Autodesk Inventor part; units mm, degrees
sketch "Sketch1" plane through (0, 0, 0) normal (0, 0, 1) x (1, 0, 0)
  line L0 (-109.5, 84.5) -> (109.5, 84.5)
  line L1 (109.5, 84.5) -> (109.5, -84.5)
  line L2 (109.5, -84.5) -> (-109.5, -84.5)
  line L3 (-109.5, -84.5) -> (-109.5, 84.5)
  point P0 (0, 84.5)
  point P1 (0, 0)
  point P2 (-109.5, 0)
  dimension "d0" = 219
  dimension "d1" = 169
extrude "Extrusion1" add sketch "Sketch1" along normal blind 6
sketch "Sketch2" plane through (0, 0, 6) normal (0, 0, 1) x (1, 0, 0)
  circle A0 centre (-103, -78) radius 3.25
  line L0 (-103, -78) -> (-103, -74) construction
  line L1 (-106.25, -68) -> (-99.75, -68)
  line L2 (-99.75, -68) -> (-99.75, -74)
  line L3 (-99.75, -74) -> (-106.25, -74)
  line L4 (-106.25, -74) -> (-106.25, -68)
  line L5 (-109.5, -84.5) -> (109.5, -84.5)
  line L6 (-109.5, -84.5) -> (-103, -84.5) construction
  line L7 (-103, -84.5) -> (-103, -78) construction
  point P0 (0, 0)
  dimension "d39" = 6.5
  dimension "d44" = 4
  dimension "d45" = 6.5
  dimension "d46" = 6
  dimension "d64" = 6.5
  dimension "d65" = 6.5
extrude "Extrusion2" cut sketch "Sketch2" against normal blind 6 contours A0
mirror "Mirror3" about plane through (0, 0, 0) normal (1, 0, 0) of "Extrusion2"
mirror "Mirror7" about plane through (0, 0, 0) normal (0, 1, 0) of "Extrusion2", "Mirror3"
sketch "Sketch7" plane through (0, 0, 6) normal (0, 0, 1) x (1, 0, 0)
  line L0 (-109.5, 84.5) -> (-109.5, -84.5)
  line L1 (-109.5, 68) -> (-75, 68)
  line L2 (-75, 68) -> (-75, -68)
  line L3 (-75, -68) -> (-109.5, -68)
  line L4 (-109.5, -68) -> (-109.5, 68)
  point P0 (0, 0)
  point P1 (-109.5, 0)
  point P2 (-109.5, 0)
  dimension "d40" = 34.5
  dimension "d41" = 136
extrude "Extrusion6" cut sketch "Sketch7" against normal blind 10
sketch "Sketch8" plane through (0, 0, 6) normal (0, 0, 1) x (1, 0, 0)
  circle A0 centre (-103, -78) radius 3.25
  line L0 (-103, -78) -> (-103, -73.75) construction
  line L1 (-106.125, -68) -> (-99.875, -68)
  line L2 (-99.875, -68) -> (-99.875, -73.75)
  line L3 (-99.875, -73.75) -> (-106.125, -73.75)
  line L4 (-106.125, -73.75) -> (-106.125, -68)
  point P0 (0, 0)
  dimension "d47" = 4.25
  dimension "d48" = 6.25
  dimension "d49" = 5.75
extrude "Extrusion7" cut sketch "Sketch8" against normal blind 6 contours L1 L2 L3 L4
mirror "Mirror8" about plane through (0, 0, 0) normal (0, 1, 0) of "Extrusion7"
fillet "Fillet5" radius 1 12 edges at (-109.5, -84.5, 3) (109.5, -84.5, 3) (-75, -68, 3) (109.5, 84.5, 3) (-109.5, 84.5, 3) (-109.5, 68, 3) (-75, 68, 3) (-99.875, 68, 3) (-106.125, 68, 3) (-99.875, -68, 3) (-109.5, -68, 3) (-106.125, -68, 3)
sketch "Sketch10" plane through (0, 0, 6) normal (0, 0, 1) x (1, 0, 0)
  line L0 (-75, 44.5) -> (39, 44.5) construction
  line L1 (39, 44.5) -> (39, -44.5) construction
  line L2 (39, -44.5) -> (-75, -44.5) construction
  line L3 (-75, -44.5) -> (-75, 44.5) construction
  line L4 (-75, 67) -> (-75, -67)
  line L5 (-75, 44.5) -> (39, -44.5) construction
  circle A0 centre (0, 0) radius 8.25
  line L6 (0, 0) -> (0, 25) construction
  circle A1 centre (0, 25) radius 8.25
  point P0 (-75, 0)
  point P1 (-75, 0)
  point P2 (-75, 0)
  dimension "d53" = 114
  dimension "d54" = 89
  dimension "d55" = 16.5
  dimension "d56" = 25
  dimension "d57" = 16.5
extrude "Extrusion8" cut sketch "Sketch10" against normal through all
pattern_circular "Circular Pattern1" count 8 over 360 about axis through (0, 0, 6) along (0, 0, -1) of "Extrusion8"
equation "\"d7\" = d46"
properties part number "MDF_Top_Big_Mic" material "MDF Medium Density Fiberboard"
Read the model definition and answer for the solid it produces. Units are mm, in the model's axes. A direction names the side the tool comes from. Coordinates: 2 decimals unless noted, no trailing zeros. Loops run counter-clockwise (first coordinate to the right, second up) from the corner with the lowest first, then second, coordinate; pieces in that order, holes last. Notation, with made-up numbers: (-2, 71.5) - (17, 71.5) arc R25 ccw to (17, 98.5) - close; hole circle Ø11 at (34.5, -31). An arc over 180 degrees is marked (long way). Answer in a Markdown table with one row per item.
1. Straight lines are drawn through the part: line 1 (Y direction, x = 0, z = 3.95); line 2 (X direction, y = 0.5, z = 2.7); line 3 (X direction, y = 11, z = 1.7). For each, find the intervals that lie inside material, in ascending order.
Conclusion:
| item | result |
|---|---|
| line 1 | y = -84.5 to -33.25, -16.75 to -8.25, 8.25 to 16.75, 33.25 to 84.5 |
| line 2 | x = -75 to -33.23, -16.77 to -8.23, 8.23 to 16.77, 33.23 to 109.5 |
| line 3 | x = -75 to -22.52, -12.83 to 12.83, 22.52 to 109.5 |
2. Given pin 1 (6 mm diameter, centred on x = 103, y = 78, fed in from +Z); pin 2 (1.8 mm diameter, centred on y = -6, z = 4.5, fed in from -X), each flat-ended and moving along its own axis, determine where each tip first touches the part or whether it passes through.
Conclusion:
| item | result |
|---|---|
| pin 1 | passes through |
| pin 2 | stops at x = -75 |
3. Determine the mould class of faces 4 (the face through (-2, 39, 6)), 5 (the face through (-99.875, 71, 3)), 6 (the face through (109.5, 1, 3)) for opening direction X: +X half, -X half, draft (parallel to the pull), parting line (faces both ways), or undercut.
Conclusion:
| item | result |
|---|---|
| face 4 | draft |
| face 5 | undercut |
| face 6 | +X half |
4. Which of the six approach directions +Z, -Z, +X, -X, +Y, -Y give full straight-line access (tool end or side, diameter ignored) to faces 1 (the face through (-75, 1, 3)), 2 (the face through (-2, 39, 0)), 3 (the face through (-99.875, -71, 3))?
Conclusion:
| item | result |
|---|---|
| face 1 | +Z, -Z, -X |
| face 2 | -Z, +X, -X, +Y, -Y |
| face 3 | +Z, -Z |
5. Find section B-B, the plane y = 0. Write down the section's boundary in (x, z).
Conclusion:
| item | result |
|---|---|
| outline | (-75, 0) - (-33.25, 0) - (-33.25, 6) - (-75, 6) - close; (-16.75, 0) - (-8.25, 0) - (-8.25, 6) - (-16.75, 6) - close; (8.25, 0) - (16.75, 0) - (16.75, 6) - (8.25, 6) - close; (33.25, 0) - (109.5, 0) - (109.5, 6) - (33.25, 6) - close |
6. Find section C-C, the plane y = 19.5. Write down the section's boundary in (x, z).
Conclusion:
| item | result |
|---|---|
| outline | (-75, 0) - (-25.72, 0) - (-25.72, 6) - (-75, 6) - close; (-9.63, 0) - (-6.15, 0) - (-6.15, 6) - (-9.63, 6) - close; (6.15, 0) - (9.63, 0) - (9.63, 6) - (6.15, 6) - close; (25.72, 0) - (109.5, 0) - (109.5, 6) - (25.72, 6) - close |
7. Find section A-A, the plane x = -85. Write down the section's boundary in (y, z), then the cut area to 3 significant figures.
Conclusion:
| item | result |
|---|---|
| outline | (-84.5, 0) - (-68, 0) - (-68, 6) - (-84.5, 6) - close; (68, 0) - (84.5, 0) - (84.5, 6) - (68, 6) - close |
| area | 198 mm² |
